```python
from build123d import *

# Parameters (mm, degrees)
EXTRUDE_1_DEPTH     = 35
RIB_1_REACH         = 59.21
SKETCH_3_WALL_W     = 154.604044108
SKETCH_3_WALL_H     = 3
CUT_EXTRUDE_1_DEPTH = 3
SKETCH_6_R          = 1.65
CUT_EXTRUDE_2_DEPTH = 8
CUT_EXTRUDE_3_DEPTH = 3
SKETCH_8_R          = 1.65
CUT_EXTRUDE_4_DEPTH = 10
FILLET_1_R          = 2


with BuildPart() as part:
    # Эскиз1 → Бобышка-Вытянуть1 (new body)
    with BuildSketch(Plane.XY):
        Polygon((0, 0), (-32, 0), (-32, 5), (-5, 5), (-5, 32), (0, 32), align=None)
    extrude(amount=EXTRUDE_1_DEPTH)

    # Эскиз3 wall → Ребро1 (add, up to next)
    with BuildSketch(Plane(origin=(-18.5, 18.5, 35), x_dir=(0.707106781187, 0.707106781187, 0), z_dir=(-0.707106781187, 0.707106781187, 0)), mode=Mode.PRIVATE) as rib_1_sk1:
        with Locations((0, 1.5)):
            Rectangle(SKETCH_3_WALL_W, SKETCH_3_WALL_H)
    rib_1_tool1 = extrude(rib_1_sk1.sketch, amount=-RIB_1_REACH, mode=Mode.PRIVATE) - part.part
    rib_1 = rib_1_tool1.solids().sort_by_distance((-18.5, 18.5, 35))[0]
    add(rib_1)

    # Зеркальное отражение1: Ребро1 across plane
    add(rib_1.mirror(Plane.XY.offset(17.5)))

    # Эскиз5 → Вырез-Вытянуть1 (cut)
    with BuildSketch(Plane.ZY.offset(5)):
        Polygon((24, 8.984174247), (27, 10.716225055), (27, 14.18032667), (24, 15.912377477), (21, 14.18032667), (21, 10.716225055), align=None)
        Polygon((11, 21.087622523), (14, 22.81967333), (14, 26.283774945), (11, 28.015825753), (8, 26.283774945), (8, 22.81967333), align=None)
    extrude(amount=-CUT_EXTRUDE_1_DEPTH, mode=Mode.SUBTRACT)

    # Эскиз6 → Вырез-Вытянуть2 (cut)
    with BuildSketch(Plane.ZY.offset(2)):
        with Locations((11, 24.551724138)):
            Circle(SKETCH_6_R)
        with Locations((24, 12.448275862)):
            Circle(SKETCH_6_R)
    extrude(amount=-CUT_EXTRUDE_2_DEPTH, mode=Mode.SUBTRACT)

    # Эскиз7 → Вырез-Вытянуть3 (cut)
    with BuildSketch(Plane(origin=(0, 5, 0), x_dir=(1, 0, 0), z_dir=(0, 1, 0))):
        Polygon((-24.551724138, -20.535898385), (-27.551724138, -22.267949192), (-27.551724138, -25.732050808), (-24.551724138, -27.464101615), (-21.551724138, -25.732050808), (-21.551724138, -22.267949192), align=None)
        Polygon((-12.448275862, -7.535898385), (-15.448275862, -9.267949192), (-15.448275862, -12.732050808), (-12.448275862, -14.464101615), (-9.448275862, -12.732050808), (-9.448275862, -9.267949192), align=None)
    extrude(amount=-CUT_EXTRUDE_3_DEPTH, mode=Mode.SUBTRACT)

    # Эскиз8 → Вырез-Вытянуть4 (cut)
    with BuildSketch(Plane(origin=(0, 2, 0), x_dir=(1, 0, 0), z_dir=(0, 1, 0))):
        with Locations(Location((-24.551724138, -24, 0), (0, 0, 270))):
            Circle(SKETCH_8_R)
        with Locations(Location((-12.448275862, -11, 0), (0, 0, 270))):
            Circle(SKETCH_8_R)
    extrude(amount=-CUT_EXTRUDE_4_DEPTH, mode=Mode.SUBTRACT)

    # Скругление1
    fillet_1_edges = [part.edges().sort_by_distance(p)[0] for p in [
        (-32, 2.5, 35),
        (-32, 2.5, 0),
        (-2.5, 32, 0),
        (-2.5, 32, 35),
    ]]
    fillet(fillet_1_edges, radius=FILLET_1_R)


solid = part.part
```
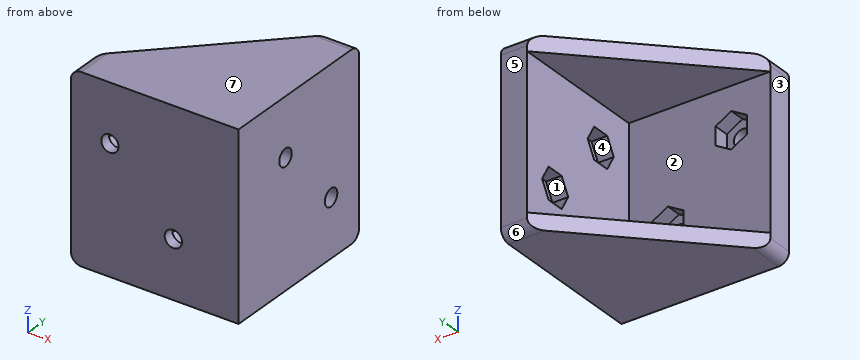
Can you work these out from the model? Positions are in its coordinate system, mm. Face numbers are marked on the shaded views. A direction names the side the tool comes from. Round coordinates to 2 decimals unless told otherwise and drop trailing zeros. Order: outer loops, then holes, each group sorted by start corner. A loop starts at its lowest first (then second) coordinate and runs counter-clockwise, first axis right, second up. Notation, with made-up numbers: (-22.5, 44) -> (-15.5, 44) arc R22 ccw to (-15.5, 63) -> close; hole circle Ø3 at (-11, 23). An arc over 180 degrees is marked (long way). Return JSON: item names as keys, results as strings. Group by question number.
1. If we section it at D-D, the plane z = 16: Write out the boundary of the cut face in (x, y), then the cut area to 3 significant figures.
2. If we section it at B-B, the plane y = 28.5: Write out the boundary of the cut face in (x, z), then the cut area to 3 significant figures.
3. If we section it at C-C, the plane x = -18: Write out the boundary of the cut face in (y, z), then the cut area to 3 significant figures.
4. Will these pins go through, and if not, where does the flat tip stop? pin 1 (8 mm diameter, centred on x = -27, z = 7.5, fed in from +Y); pin 2 (6.5 mm diameter, centred on y = 13, z = 25, fed in from -X).
5. Which directions (+Z, -Z, +X, -X, +Y, -Y) give clear straight access to the entire face, cutting with the end or side of a thin tool? Please do the marked faces 1, 2 and 3.
6. We'd pull the mould along Z, two halves only. Please class the marked faces 4, 5, 6 and 7: released by +Z, released by -Z, zero draft, split by the parting line, or undercut.
7. If we section it at A-A, the plane x = -3: Write out the boundary of the cut face in (y, z).
8. I need wall thicknesses on line 1 (Z direction, x = -24, y = 11); line 2 (X direction, y = 1.1, z = 11); line 3 (Y direction, x = -1.25, z = 24). Which ranges of each line are inside material? Lowest first, please. Write a range as [from, to].
Output values:
{
 "1": {"outline": "(-32, 0) -> (0, 0) -> (0, 32) -> (-5, 32) -> (-5, 5) -> (-32, 5) -> close", "area": "295 mm²"},
 "2": {"outline": "(-8.5, 0) -> (0, 0) -> (0, 35) -> (-8.5, 35) -> (-8.5, 32) -> (-5, 32) -> (-5, 3) -> (-8.5, 3) -> close", "area": "196 mm²"},
 "3": {"outline": "(0, 0) -> (19, 0) -> (19, 3) -> (5, 3) -> (5, 32) -> (19, 32) -> (19, 35) -> (0, 35) -> close", "area": "259 mm²"},
 "4": {"pin 1": "y = 5", "pin 2": "x = -5"},
 "5": {"face 1": "-X", "face 2": "-X, +Y", "face 3": "+Z, -Z, -X, +Y, -Y"},
 "6": {"face 4": "undercut", "face 5": "zero draft", "face 6": "released by -Z", "face 7": "released by +Z"},
 "7": {"outline": "(0, 0) -> (30, 0) arc R2 ccw to (32, 2) -> (32, 33) arc R2 ccw to (30, 35) -> (0, 35) -> close; hole (8.98, 24) -> (10.72, 21) -> (14.18, 21) -> (15.91, 24) -> (14.18, 27) -> (10.72, 27) -> close; hole (21.09, 11) -> (22.82, 8) -> (26.28, 8) -> (28.02, 11) -> (26.28, 14) -> (22.82, 14) -> close"},
 "8": {"line 1": "[0, 3], [32, 35]", "line 2": "[-32, -14.1], [-10.8, 0]", "line 3": "[0, 10.8], [14.1, 32]"}
}
